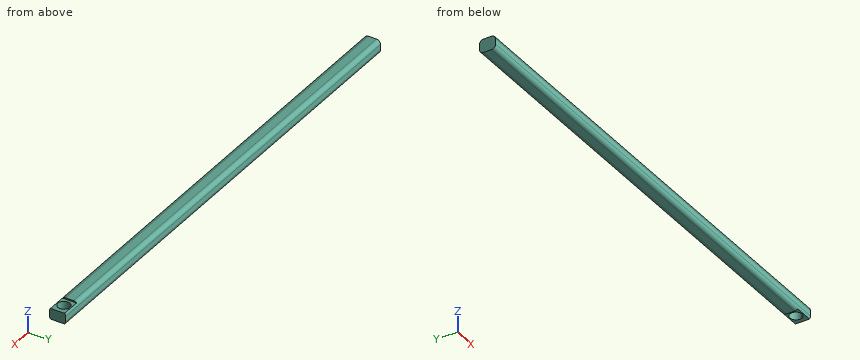
from build123d import *

# Parameters (mm, degrees)
CROQUIS1_W                 = 37.5
CROQUIS1_H                 = 30
SALIENTE_EXTRUIR1_DEPTH    = 15
CROQUIS2_R                 = 2.1
SALIENTE_EXTRUIR2_DEPTH    = 1
SALIENTE_EXTRUIR3_DEPTH    = 35
CROQUIS5_W                 = 18
CROQUIS5_H                 = 12
CROQUIS5_R                 = 4.5
SALIENTE_EXTRUIR4_DEPTH    = 5
CROQUIS6_W                 = 1
CROQUIS6_H                 = 12
CORTAR_EXTRUIR2_DEPTH      = 14
REDONDEO2_R                = 3
CORTAR_EXTRUIR3_DEPTH      = 78.447159406
CORTAR_EXTRUIR3_DEPTH_BACK = 78.447159406
CROQUIS7_OUTSIDE_W         = 123.972
CROQUIS7_OUTSIDE_H         = 74.472
CROQUIS7_OUTSIDE_W_2       = 24.163279834
CROQUIS7_OUTSIDE_H_2       = 36.211204922
SALIENTE_EXTRUIR5_DEPTH    = 350


with BuildPart() as part:
    # Croquis1 → Saliente-Extruir1 (new body)
    with BuildSketch(Plane.XY):
        Rectangle(CROQUIS1_W, CROQUIS1_H)
    extrude(amount=SALIENTE_EXTRUIR1_DEPTH)

    # Croquis2 → Saliente-Extruir2 (add)
    # profile 1 of 3: a face of its own
    with BuildSketch(Plane.XY):
        with BuildLine():
            Line((-18.75, 3.7), (-26.75, 3.7))
            ThreePointArc((-26.75, 3.7), (-27.457106781, 3.407106781), (-27.75, 2.7))
            Line((-27.75, 2.7), (-27.75, -2.7))
            ThreePointArc((-27.75, -2.7), (-27.457106781, -3.407106781), (-26.75, -3.7))
            Line((-26.75, -3.7), (-18.75, -3.7))
            Line((-18.75, -3.7), (-18.75, 3.7))
        make_face()
        with Locations((-23.25, 0)):
            Circle(CROQUIS2_R, mode=Mode.SUBTRACT)
    # profile 2 of 3: a face of its own
    with BuildSketch(Plane.XY):
        with BuildLine():
            Line((-10, 15), (10, 15))
            Line((10, 15), (10, 24))
            ThreePointArc((10, 24), (9.707106781, 24.707106781), (9, 25))
            Line((9, 25), (-9, 25))
            ThreePointArc((-9, 25), (-9.707106781, 24.707106781), (-10, 24))
            Line((-10, 24), (-10, 15))
        make_face()
        with Locations((-5.5, 20)):
            Circle(CROQUIS2_R, mode=Mode.SUBTRACT)
        with Locations((5.5, 20)):
            Circle(CROQUIS2_R, mode=Mode.SUBTRACT)
    # profile 3 of 3: a face of its own
    with BuildSketch(Plane.XY):
        with BuildLine():
            Line((-9, -25), (9, -25))
            ThreePointArc((9, -25), (9.707106781, -24.707106781), (10, -24))
            Line((10, -24), (10, -15))
            Line((10, -15), (-10, -15))
            Line((-10, -15), (-10, -24))
            ThreePointArc((-10, -24), (-9.707106781, -24.707106781), (-9, -25))
        make_face()
        with Locations(Location((5.5, -20, 0), (0, 0, 180))):
            Circle(CROQUIS2_R, mode=Mode.SUBTRACT)
        with Locations(Location((-5.5, -20, 0), (0, 0, 180))):
            Circle(CROQUIS2_R, mode=Mode.SUBTRACT)
    extrude(amount=SALIENTE_EXTRUIR2_DEPTH)

    # Croquis3 → Saliente-Extruir3 (add)
    with BuildSketch(Plane(origin=(18.75, 0, 0), x_dir=(0, 0, -1), z_dir=(1, 0, 0))):
        with BuildLine():
            Line((-10.5, -12.5), (-4.5, -12.5))
            ThreePointArc((-4.5, -12.5), (-2.378679656, -11.621320344), (-1.5, -9.5))
            Line((-1.5, -9.5), (-1.5, 9.5))
            ThreePointArc((-1.5, 9.5), (-2.378679656, 11.621320344), (-4.5, 12.5))
            Line((-4.5, 12.5), (-10.5, 12.5))
            ThreePointArc((-10.5, 12.5), (-12.621320344, 11.621320344), (-13.5, 9.5))
            Line((-13.5, 9.5), (-13.5, -9.5))
            ThreePointArc((-13.5, -9.5), (-12.621320344, -11.621320344), (-10.5, -12.5))
        make_face()
    extrude(amount=SALIENTE_EXTRUIR3_DEPTH)

    # Croquis5 → Saliente-Extruir4 (add, symmetric)
    with BuildSketch(Plane.XY.offset(7.5)):
        with Locations((62.75, 0)):
            Rectangle(CROQUIS5_W, CROQUIS5_H)
        with Locations((64.25, 0)):
            Circle(CROQUIS5_R, mode=Mode.SUBTRACT)
    extrude(amount=SALIENTE_EXTRUIR4_DEPTH, both=True)

    # Croquis6 → Cortar-Extruir2 (cut)
    with BuildSketch(Plane(origin=(71.75, 0, 0), x_dir=(0, 0, -1), z_dir=(1, 0, 0))):
        with Locations((-12, 0)):
            Rectangle(CROQUIS6_W, CROQUIS6_H)
        with Locations((-3, 0)):
            Rectangle(CROQUIS6_W, CROQUIS6_H)
    extrude(amount=-CORTAR_EXTRUIR2_DEPTH, mode=Mode.SUBTRACT)

    # Redondeo2
    redondeo2_edges = [part.edges().sort_by_distance(p)[0] for p in [
        (55.75, -6, 12.5),
        (55.75, -6, 2.5),
        (55.75, 6, 2.5),
        (55.75, 6, 12.5),
    ]]
    fillet(redondeo2_edges, radius=REDONDEO2_R)

    # Croquis7 outside → Cortar-Extruir3 (cut, two sides: drawn at the far end of the back side and taken through both)
    with BuildSketch(Plane.XY.offset(15).offset(-CORTAR_EXTRUIR3_DEPTH_BACK)):
        with Locations((22, 0)):
            Rectangle(CROQUIS7_OUTSIDE_W, CROQUIS7_OUTSIDE_H)
        with Locations((65.831639917, -3.105602461)):
            Rectangle(CROQUIS7_OUTSIDE_W_2, CROQUIS7_OUTSIDE_H_2, mode=Mode.SUBTRACT)
    extrude(amount=CORTAR_EXTRUIR3_DEPTH + CORTAR_EXTRUIR3_DEPTH_BACK, mode=Mode.SUBTRACT)

    # Croquis10 → Saliente-Extruir5 (add)
    with BuildSketch(Plane.ZY.offset(-53.75)):
        with BuildLine():
            Line((5.5, -6), (9.5, -6))
            ThreePointArc((9.5, -6), (11.621320344, -5.121320344), (12.5, -3))
            Line((12.5, -3), (12.5, 3))
            ThreePointArc((12.5, 3), (11.621320344, 5.121320344), (9.5, 6))
            Line((9.5, 6), (5.5, 6))
            ThreePointArc((5.5, 6), (3.378679656, 5.121320344), (2.5, 3))
            Line((2.5, 3), (2.5, -3))
            ThreePointArc((2.5, -3), (3.378679656, -5.121320344), (5.5, -6))
        make_face()
    extrude(amount=SALIENTE_EXTRUIR5_DEPTH)


solid = part.part
Check sheet for the modelled part. Datum: model origin and axes. Units: mm. Coordinates: 2 decimals unless noted, no trailing zeros. Loops run counter-clockwise (first coordinate to the right, second up) from the corner with the lowest first, then second, coordinate; pieces in that order, holes last. Notation, with made-up numbers: (-5, -32.75) -> (9, -32.75) arc R17 ccw to (9, -5.75) -> close; hole circle Ø7 at (89, 71). An arc over 180 degrees is marked (long way). Write item = value, one per line. Start each with the question number.
1. Section check C-C on x = -205. Record the cut outline in (y, z), then the cut area to 3 significant figures.
2. Section check B-B on x = 64.25. Record the cut outline in (y, z).
3. Section check A-A on y = 0. Record the cut outline in (x, z).
4. Depth check by flat-ended pin: P1, Ø5, axis at x = 67, y = 1.5, coming from the -Z side; P2, Ø5, axis at x = 65.5, y = 2, coming from the +Z side. Enter the tip coordinate at first touch or a pass-through.
5. Material ranges on line 1 (X direction, y = 0, z = 6); line 2 (Y direction, x = 64.25, z = 6.5); line 3 (Y direction, x = -25, z = 5), recorded low to high.
Responses:
q1.outline = (-6, 5.5) arc R3 ccw to (-3, 2.5) -> (3, 2.5) arc R3 ccw to (6, 5.5) -> (6, 9.5) arc R3 ccw to (3, 12.5) -> (-3, 12.5) arc R3 ccw to (-6, 9.5) -> close
q1.area = 112 mm2
q2.outline = (-6, 5.5) arc R3 ccw to (-5.24, 3.5) -> (-4.5, 3.5) -> (-4.5, 11.5) -> (-5.24, 11.5) arc R3 ccw to (-6, 9.5) -> close; (4.5, 3.5) -> (5.24, 3.5) arc R3 ccw to (6, 5.5) -> (6, 9.5) arc R3 ccw to (5.24, 11.5) -> (4.5, 11.5) -> close
q3.outline = (-296.25, 2.5) -> (57.75, 2.5) -> (57.75, 3.5) -> (59.75, 3.5) -> (59.75, 11.5) -> (57.75, 11.5) -> (57.75, 12.5) -> (-296.25, 12.5) -> close; (68.75, 3.5) -> (71.75, 3.5) -> (71.75, 11.5) -> (68.75, 11.5) -> close
q4.P1 = 3.5
q4.P2 = 11.5
q5.line_1 = -296.25 to 59.75, 68.75 to 71.75
q5.line_2 = -6 to -4.5, 4.5 to 6
q5.line_3 = -5.96 to 5.96
